Geometry check sheet. Reference: the model listing, model coordinates, mm. A direction names the side the tool comes from. Round coordinates to 2 decimals unless told otherwise and drop trailing zeros. Order: outer loops, then holes, each group sorted by start corner. A loop starts at its lowest first (then second) coordinate and runs counter-clockwise, first axis right, second up. Notation, with made-up numbers: (-8.5, 13.5) - (2.5, 13.5) arc R25 cw to (2.5, 35.5) - close; hole circle Ø5 at (41, -5.5). An arc over 180 degrees is marked (long way). Use a Markdown table: item, result. Add a question column.
(1) Section check B-B on x = 74.5. Record the boundary of the cut face in (y, z), then the cut area to 3 significant figures.
(2) Thickness scan on line 1 along Z through (x, y) = (77, -1); line 2 along Z through (x, y) = (0, 80). Record the ranges inside material, lowest first. Write a range as [from, to].
(3) Section check A-A on z = 0. Record the boundary of the cut face in (x, y), then the cut area to 3 significant figures.
(4) Access from +Z, -Z, +X, -X, +Y, -Y to the whole of each face (thin tool, end or side, straight path). Record for faces 5 (the face through (101.6, 43, -14)), 6 (the face through (73.425, 13.352, -42.397)), 7 (the face through (42.397, 70.117, -13.352)).
(5) Mould release check, pull along Z, two halves, no side actions. Record for faces 1 (the face through (46.03, 69.58, 14.5)), 2 (the face through (44.45, -36, -13)), 3 (the face through (33, 50.8, -20)), 4 (the face through (-14, 88.9, 43)): released by +Z, released by -Z, zero draft, split by the parting line, or undercut.
(6) Gauge pin test, flat ends, axial feed: P1, Ø3, axis at x = 75, z = -25.5, coming from the +Y side; P2, Ø1, axis at x = 2.5, y = 14.5, coming from the +Z side; P3, Ø2, axis at x = 38, z = -16, coming from the +Y side. Record the tip position at first contact, or that the pin passes through.
(7) Section check C-C on z = 31. Record the boundary of the cut face in (x, y), then the cut area to 3 significant figures.
```python
from build123d import *

# Parameters (mm, degrees)
SKETCH2_R          = 48.26
SKETCH2_R_2        = 38.1
SKETCH3_R          = 44.45
SKETCH3_R_2        = 38.1
CUT_EXTRUDE1_DEPTH = 57.15
SKETCH4_R          = 44.45
SKETCH4_R_2        = 38.1
CUT_EXTRUDE2_DEPTH = 38.1


with BuildPart() as part:
    # Sweep1: sweep along a path in Sketch1
    with BuildLine(Plane.XY) as sweep1_path:
        Line((0, 88.9), (0, 50.8))
        ThreePointArc((0, 50.8), (14.878975516, 14.878975516), (50.8, 0))
        Line((50.8, 0), (101.6, 0))
    # Sketch2 → Sweep1 (sweep)
    with BuildSketch(Plane(origin=(0, 88.9, 0), x_dir=(1, 0, 0), z_dir=(0, 1, 0))):
        Circle(SKETCH2_R)
        Circle(SKETCH2_R_2, mode=Mode.SUBTRACT)
    sweep(path=sweep1_path.line)

    # Sketch3 → Cut-Extrude1 (cut)
    with BuildSketch(Plane(origin=(101.6, 0, 0), x_dir=(0, 0, -1), z_dir=(1, 0, 0))):
        Circle(SKETCH3_R)
        Circle(SKETCH3_R_2, mode=Mode.SUBTRACT)
    extrude(amount=-CUT_EXTRUDE1_DEPTH, mode=Mode.SUBTRACT)

    # Sketch4 → Cut-Extrude2 (cut)
    with BuildSketch(Plane(origin=(0, 88.9, 0), x_dir=(1, 0, 0), z_dir=(0, 1, 0))):
        Circle(SKETCH4_R)
        Circle(SKETCH4_R_2, mode=Mode.SUBTRACT)
    extrude(amount=-CUT_EXTRUDE2_DEPTH, mode=Mode.SUBTRACT)


solid = part.part
```
Check sheet entries:
| question | item | result |
|---|---|---|
| 1 | outline | circle Ø96.52 at (0, 0); hole circle Ø88.9 at (0, 0) |
| 1 | area | 1,110 mm2 |
| 2 | line 1 | z = [-48.25, -44.44], [44.44, 48.25] |
| 2 | line 2 | z = [-48.26, -44.45], [44.45, 48.26] |
| 3 | outline | (-48.26, 50.8) arc R99.06 ccw to (50.8, -48.26) - (101.6, -48.26) - (101.6, -44.45) - (44.45, -44.45) - (44.45, -38.1) - (50.8, -38.1) arc R88.9 cw to (-38.1, 50.8) - (-44.45, 50.8) - (-44.45, 88.9) - (-48.26, 88.9) - close; (38.1, 50.8) arc R12.7 ccw to (44.45, 39.8) - (44.45, 44.45) - (101.6, 44.45) - (101.6, 48.26) - (50.8, 48.26) arc R2.54 cw to (48.26, 50.8) - (48.26, 88.9) - (44.45, 88.9) - (44.45, 50.8) - close |
| 3 | area | 2,220 mm2 |
| 4 | face 5 | +Z, -Z, +X, +Y, -Y |
| 4 | face 6 | +X |
| 4 | face 7 | +Y |
| 5 | face 1 | split by the parting line |
| 5 | face 2 | undercut |
| 5 | face 3 | undercut |
| 5 | face 4 | zero draft |
| 6 | P1 | stops at y = 41.87 |
| 6 | P2 | stops at z = 47.39 |
| 6 | P3 | stops at y = 50.8 |
| 7 | outline | (-36.99, 50.8) arc R87.79 ccw to (50.8, -36.99) - (101.6, -36.99) - (101.6, -31.86) - (44.45, -31.86) - (44.45, -22.15) - (50.8, -22.15) arc R72.95 cw to (-22.15, 50.8) - (-31.86, 50.8) - (-31.86, 88.9) - (-36.99, 88.9) - close; (22.15, 50.8) arc R28.65 ccw to (44.45, 22.86) - (44.45, 31.86) - (101.6, 31.86) - (101.6, 36.99) - (50.8, 36.99) arc R13.81 cw to (36.99, 50.8) - (36.99, 88.9) - (31.86, 88.9) - (31.86, 50.8) - close |
| 7 | area | 3,160 mm2 |
